Source: three-view drawing plus pictorial views. Frame: mm from the lowest corner of the part. Give positions to 0.01 mm unless a question says otherwise; leave off trailing zeros. Loops run counter-clockwise (first coordinate to the right, second up) from the corner with the lowest first, then second, coordinate; pieces in that order, holes last. Notation, with made-up numbers: (25, -3.5) - (47, -3.5) arc R18 cw to (47, 8.5) - close; hole circle Ø10 at (-39, 78). An arc over 180 degrees is marked (long way). Answer in a Markdown table with one row per item.
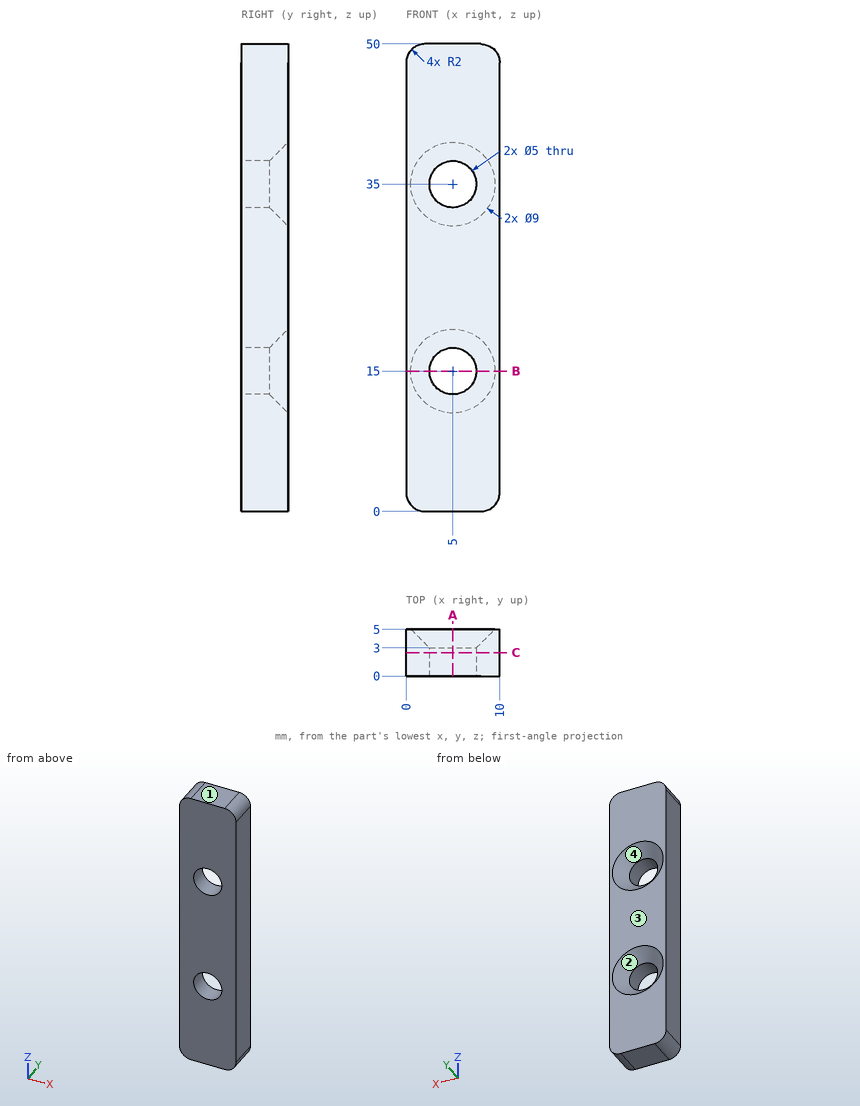
Q1. Cut plane C-C (y = 2.5). Output: boundary loops of the cut face in (x, z), and give its area (3 significant figures).
Check values:
| item | result |
|---|---|
| outline | (0, 2) arc R2 ccw to (2, 0) - (8, 0) arc R2 ccw to (10, 2) - (10, 48) arc R2 ccw to (8, 50) - (2, 50) arc R2 ccw to (0, 48) - close; hole circle Ø5 at (5, 15); hole circle Ø5 at (5, 35) |
| area | 457 mm² |
Q2. First-contact query: pin 1 (3 mm diameter, centred on x = 5, z = 35, fed in from -Y). Flat tip, straight axial feed; report the tip coordinate or a pass-through.
Check values:
| item | result |
|---|---|
| pin 1 | through |
Q3. Material intervals for line 1 along Z through (x, y) = (5, 2.35); line 2 along Z through (x, y) = (8.25, 4.75); line 3 along X through (y, z) = (0.8, 14.5), sorted ascending.
Check values:
| item | result |
|---|---|
| line 1 | 0 to 12.5, 17.5 to 32.5, 37.5 to 50 |
| line 2 | 0.02 to 12.26, 17.74 to 32.26, 37.74 to 49.98 |
| line 3 | 0 to 2.55, 7.45 to 10 |
Q4. Draft query along Z for the marked faces 1, 2, 3 and 4. Return one class per face: pulls with the +Z half, pulls with the -Z half, needs draft (parallel to the pull), parting line crosses it, or undercut.
Check values:
| item | result |
|---|---|
| face 1 | pulls with the +Z half |
| face 2 | undercut |
| face 3 | needs draft |
| face 4 | undercut |
Q5. Cut plane A-A (x = 5). Output: boundary loops of the cut face in (y, z), and give its area (3 significant figures).
Check values:
| item | result |
|---|---|
| outline | (0, 0) - (5, 0) - (5, 10.5) - (3, 12.5) - (0, 12.5) - close; (0, 17.5) - (3, 17.5) - (5, 19.5) - (5, 30.5) - (3, 32.5) - (0, 32.5) - close; (0, 37.5) - (3, 37.5) - (5, 39.5) - (5, 50) - (0, 50) - close |
| area | 192 mm² |
Q6. Cut plane B-B (z = 15). Output: boundary loops of the cut face in (x, y), and give its area (3 significant figures).
Check values:
| item | result |
|---|---|
| outline | (0, 0) - (2.5, 0) - (2.5, 3) - (0.5, 5) - (0, 5) - close; (7.5, 0) - (10, 0) - (10, 5) - (9.5, 5) - (7.5, 3) - close |
| area | 21.0 mm² |
